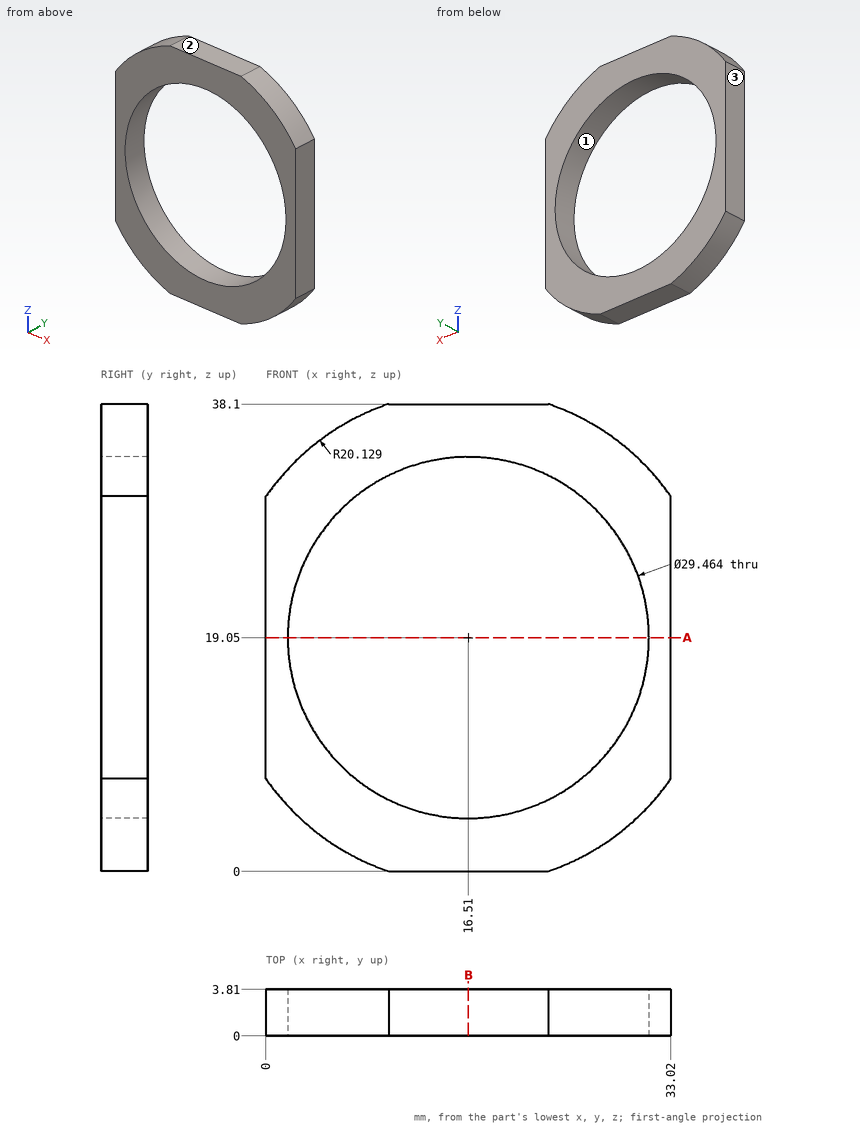
Can you work these out from the drawing? Everything is in mm from the part's minimum corner. Coordinates: 2 decimals unless noted, no trailing zeros. Write each loop counter-clockwise with the first axis right and the second up, starting at its lowest first coordinate (ties: lowest second). Pieces come first, ordered by that corner, then holes. Notation, with made-up numbers: (66.25, 43.25) - (73.25, 43.25) arc R20 ccw to (73.25, 50.25) - close; hole circle Ø1 at (64.5, 64). An arc over 180 degrees is marked (long way). Use a Markdown table: item, result.
Q1. Imagine slicing it at A-A (z = 19.05). List the corners of the cut face in (x, y) for me.
Geometry check:
| item | result |
|---|---|
| outline | (0, 0) - (1.78, 0) - (1.78, 3.81) - (0, 3.81) - close; (31.24, 0) - (33.02, 0) - (33.02, 3.81) - (31.24, 3.81) - close |
Q2. I'm going to push flat-ended pins straight in: pin 1 Ø1.5 at (x, y) = (25, 2.5) entering from -Z; pin 2 Ø10 at (x, z) = (15, 29.5) entering from -Y. Where does each tip first touch, or does it pass through?
Geometry check:
| item | result |
|---|---|
| pin 1 | stops at z = 0.47 |
| pin 2 | stops at y = 0 |
Q3. Imagine slicing it at B-B (x = 16.51). List the corners of the cut face in (y, z) for me.
Geometry check:
| item | result |
|---|---|
| outline | (0, 0) - (3.81, 0) - (3.81, 4.32) - (0, 4.32) - close; (0, 33.78) - (3.81, 33.78) - (3.81, 38.1) - (0, 38.1) - close |
Q4. Please list where these lines run through material, in increasing order: L1, parallel to Z at x = 16.51, y = 2.85; L2, parallel to X at y = 2.3, z = 16; L3, parallel to Z at x = 20, y = 3.55.
Geometry check:
| item | result |
|---|---|
| L1 | z = 0 to 4.32, 33.78 to 38.1 |
| L2 | x = 0 to 2.1, 30.92 to 33.02 |
| L3 | z = 0 to 4.74, 33.36 to 38.1 |
Q5. Thinking about a two-plate mould opening in Z: for the marked faces 1, 2 and 3, which applies, +Z half, -Z half, draft (parallel to the pull), parting line (faces both ways), or undercut?
Geometry check:
| item | result |
|---|---|
| face 1 | undercut |
| face 2 | +Z half |
| face 3 | draft |
